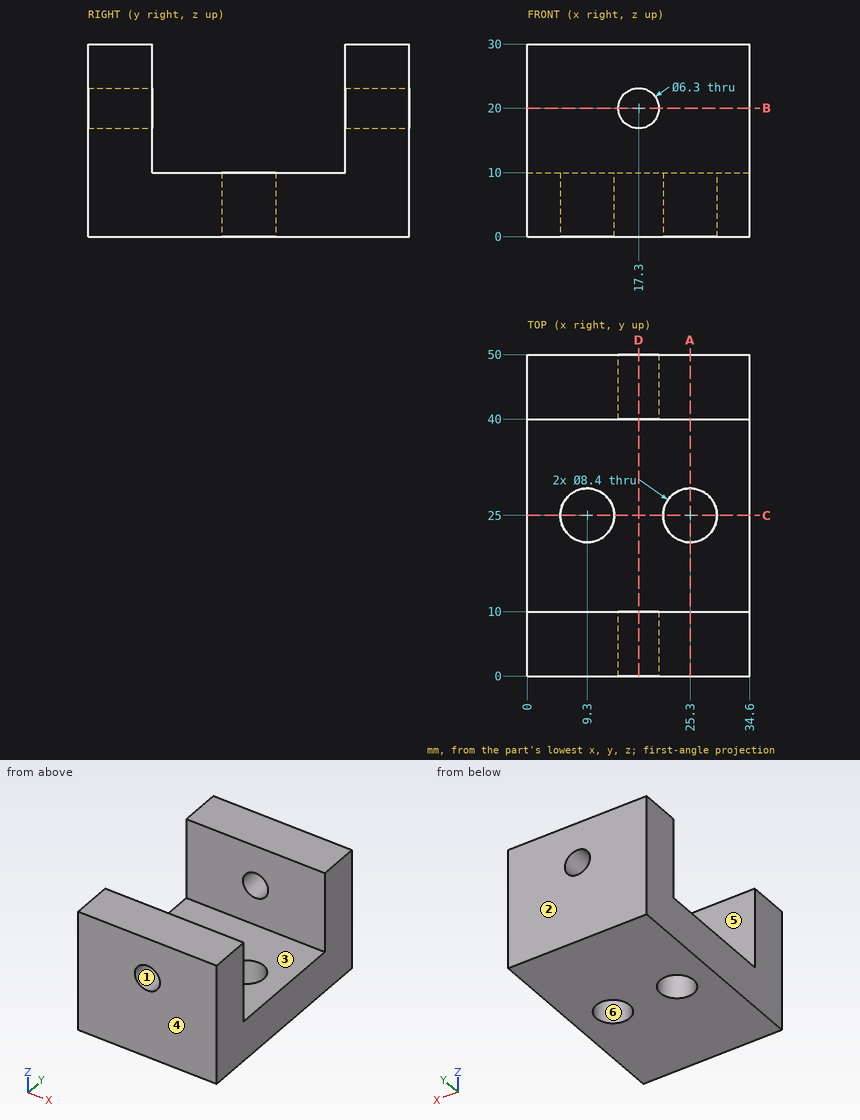
Geometry check sheet. Reference: drawing and pictorial views, mm from the part's lowest x, y, z. A direction names the side the tool comes from. Give positions to 0.01 mm unless a question says otherwise; leave off trailing zeros. Order: outer loops, then holes, each group sorted by start corner. A loop starts at its lowest first (then second) coordinate and runs counter-clockwise, first axis right, second up. Notation, with made-up numbers: M 16,38.25 L 23,38.25 A22 cw 23,72.25 Z; hole C -3.5,5 d3. An arc over 180 degrees is marked long. Answer as a JSON object with one key per item and string values. Group by question number.
1) Cross-section at C-C (y = 25). Enter the section's corners in (x, z), then the cut area to 3 significant figures.
2) Access from +Z, -Z, +X, -X, +Y, -Y to the whole of each face (thin tool, end or side, straight path). Record for the marked faces 5 and 6.
3) Scan lines: line 1 along X through (y, z) = (25, 5.75); line 2 along X through (y, z) = (45.5, 20); line 3 along Y through (x, z) = (24.5, 27.25). Record each from-to range of solid material in increasing order. Write a range as [from, to].
4) Mould release check, pull along Y, two halves, no side actions. Record for the marked faces 1, 2, 3 and 4: released by +Y, released by -Y, zero draft, split by the parting line, or undercut.
5) Cross-section at B-B (z = 20). Enter the section's corners in (x, y).
6) Cross-section at D-D (x = 17.3). Enter the section's corners in (y, z).
7) Cross-section at A-A (x = 25.3). Enter the section's corners in (y, z).
8) Depth check by flat-ended pin: pin 1 Ø6.5 at (x, y) = (9.3, 25) entering from -Z; pin 2 Ø2 at (x, y) = (5, 37) entering from +Z. Enter the tip coordinate at first touch or a pass-through.
Result sheet:
{
 "1": {"outline": "M 0,0 L 5.1,0 L 5.1,10 L 0,10 Z; M 13.5,0 L 21.1,0 L 21.1,10 L 13.5,10 Z; M 29.5,0 L 34.6,0 L 34.6,10 L 29.5,10 Z", "area": "178 mm2"},
 "2": {"face 5": "+Z, +X, -X", "face 6": "+Z, -Z"},
 "3": {"line 1": "x = [0, 5.1], [13.5, 21.1], [29.5, 34.6]", "line 2": "x = [0, 14.15], [20.45, 34.6]", "line 3": "y = [0, 10], [40, 50]"},
 "4": {"face 1": "zero draft", "face 2": "released by +Y", "face 3": "undercut", "face 4": "released by -Y"},
 "5": {"outline": "M 0,0 L 14.15,0 L 14.15,10 L 0,10 Z; M 0,40 L 14.15,40 L 14.15,50 L 0,50 Z; M 20.45,0 L 34.6,0 L 34.6,10 L 20.45,10 Z; M 20.45,40 L 34.6,40 L 34.6,50 L 20.45,50 Z"},
 "6": {"outline": "M 0,0 L 50,0 L 50,16.85 L 40,16.85 L 40,10 L 10,10 L 10,16.85 L 0,16.85 Z; M 0,23.15 L 10,23.15 L 10,30 L 0,30 Z; M 40,23.15 L 50,23.15 L 50,30 L 40,30 Z"},
 "7": {"outline": "M 0,0 L 20.8,0 L 20.8,10 L 10,10 L 10,30 L 0,30 Z; M 29.2,0 L 50,0 L 50,30 L 40,30 L 40,10 L 29.2,10 Z"},
 "8": {"pin 1": "passes through", "pin 2": "stops at z = 10"}
}
